Geometry: final body of the model. Coordinates: model frame, mm. A direction names the side the tool comes from. Give positions to 0.01 mm unless a question says otherwise; leave off trailing zeros. Write each loop counter-clockwise with the first axis right and the second up, starting at its lowest first coordinate (ties: lowest second). Pieces come first, ordered by that corner, then holes. Notation, with made-up numbers: M -37.5,-1 L -3.5,-1 A4 ccw -3.5,4 Z; hole C 53.5,-21.75 d1. An arc over 180 degrees is marked long. One line per question, with ' | ' between items.
from build123d import *

# Parameters (mm, degrees)
SKETCH1_W                   = 95.25
SKETCH1_H                   = 15
BOSS_EXTRUDE1_DEPTH         = 5
SKETCH2_W                   = 3
SKETCH2_H                   = 25.4
BOSS_EXTRUDE2_DEPTH         = 15
F_1_4_CLEARANCE_HOLE1_D     = 6.7564
F_1_4_CLEARANCE_HOLE1_DEPTH = 12
F_1_4_CLEARANCE_HOLE1_TIP   = 2.029827343
M3_CLEARANCE_HOLE1_D        = 3.6
M3_CLEARANCE_HOLE1_DEPTH    = 12
M3_CLEARANCE_HOLE1_TIP      = 1.081549114
CUT_EXTRUDE1_START          = -3
SKETCH9_R                   = 1.8
CUT_EXTRUDE1_DEPTH          = 3
FILLET1_R                   = 2
CHAMFER1_SIZE               = 1
CHAMFER2_SIZE               = 5
SKETCH10_W                  = 79.639400705
SKETCH10_H                  = 33.458041781
CUT_EXTRUDE2_DEPTH          = 57.020537529


with BuildPart() as part:
    # Sketch1 → Boss-Extrude1 (new body)
    with BuildSketch(Plane(origin=(0, 0, 0), x_dir=(1, 0, 0), z_dir=(0, 1, 0))):
        Rectangle(SKETCH1_W, SKETCH1_H)
    extrude(amount=BOSS_EXTRUDE1_DEPTH)

    # Sketch2 → Boss-Extrude2 (add, through all)
    with BuildSketch(Plane.XY.offset(7.5)):
        with Locations((-46.125, 12.7)):
            Rectangle(SKETCH2_W, SKETCH2_H)
    extrude(amount=-BOSS_EXTRUDE2_DEPTH)

    # 1/4 Clearance Hole1
    with Locations(Plane(origin=(-44.625, 0, 0), x_dir=(0, 0, -1), z_dir=(1, 0, 0))):
        with Locations((0, 12.7)):
            Hole(F_1_4_CLEARANCE_HOLE1_D / 2, depth=F_1_4_CLEARANCE_HOLE1_DEPTH)
            with Locations((0, 0, -(F_1_4_CLEARANCE_HOLE1_DEPTH + F_1_4_CLEARANCE_HOLE1_TIP / 2))):  # 118° drill point
                Cone(0, F_1_4_CLEARANCE_HOLE1_D / 2, F_1_4_CLEARANCE_HOLE1_TIP, mode=Mode.SUBTRACT)

    # M3 Clearance Hole1
    with Locations(Plane(origin=(0, 5, 0), x_dir=(1, 0, 0), z_dir=(0, 1, 0))):
        with Locations((-25, 0), (0, 0)):
            Hole(M3_CLEARANCE_HOLE1_D / 2, depth=M3_CLEARANCE_HOLE1_DEPTH)
            with Locations((0, 0, -(M3_CLEARANCE_HOLE1_DEPTH + M3_CLEARANCE_HOLE1_TIP / 2))):  # 118° drill point
                Cone(0, M3_CLEARANCE_HOLE1_D / 2, M3_CLEARANCE_HOLE1_TIP, mode=Mode.SUBTRACT)

    # Sketch9 → Cut-Extrude1 (cut)
    # profile 1 of 2: a face of its own
    with BuildSketch(Plane(origin=(0, 5, 0), x_dir=(1, 0, 0), z_dir=(0, 1, 0)).offset(CUT_EXTRUDE1_START)):
        with BuildLine():
            ThreePointArc((-26.670329309, -4.5), (-29.8, 0), (-26.670329309, 4.5))
            Line((-26.670329309, 4.5), (-41.625, 4.5))
            Line((-41.625, 4.5), (-41.625, -4.5))
            Line((-41.625, -4.5), (-26.670329309, -4.5))
        make_face()
    # profile 2 of 2: a face of its own
    with BuildSketch(Plane(origin=(0, 5, 0), x_dir=(1, 0, 0), z_dir=(0, 1, 0)).offset(CUT_EXTRUDE1_START)):
        with BuildLine():
            Line((44.625, -4.5), (44.625, 4.5))
            Line((44.625, 4.5), (-23.329670691, 4.5))
            ThreePointArc((-23.329670691, 4.5), (-21.059341382, 2.740658618), (-20.2, 0))
            ThreePointArc((-20.2, 0), (-21.059341382, -2.740658618), (-23.329670691, -4.5))
            Line((-23.329670691, -4.5), (44.625, -4.5))
        make_face()
        with Locations(Location((0, 0, 0), (0, 0, 270))):
            Circle(SKETCH9_R, mode=Mode.SUBTRACT)
    extrude(amount=CUT_EXTRUDE1_DEPTH, mode=Mode.SUBTRACT)

    # Fillet1
    fillet1_edges = [part.edges().sort_by_distance(p)[0] for p in [
        (-26.670329309, 3.5, -4.5),
        (-26.670329309, 3.5, 4.5),
        (-41.625, 3.5, 4.5),
        (-41.625, 3.5, -4.5),
        (-23.329670691, 3.5, 4.5),
        (-23.329670691, 3.5, -4.5),
    ]]
    fillet(fillet1_edges, radius=FILLET1_R)

    # Chamfer1
    chamfer1_edges = [part.edges().sort_by_distance(p)[0] for p in [
        (-44.625, 5, 0),
    ]]
    chamfer(chamfer1_edges, length=CHAMFER1_SIZE)

    # Chamfer2
    chamfer2_edges = [part.edges().sort_by_distance(p)[0] for p in [
        (-46.125, 25.4, 7.5),
        (-46.125, 25.4, -7.5),
    ]]
    chamfer(chamfer2_edges, length=CHAMFER2_SIZE)

    # Sketch10 → Cut-Extrude2 (cut, through all)
    with BuildSketch(Plane.XY.offset(7.5)):
        with Locations((39.819700352, 16.72902089)):
            Rectangle(SKETCH10_W, SKETCH10_H)
    extrude(amount=-CUT_EXTRUDE2_DEPTH, mode=Mode.SUBTRACT)

    # Mirror2: part across plane


with BuildPart() as part_1:
    add(part.part)
    add(part.part.mirror(Plane(origin=(0, 0, 0), x_dir=(0, 0, 1), z_dir=(1, 0, 0))))


solid = part_1.part
(1) Set-up query: faces 1 (the face through (-20, 4, 4)), 2 (the face through (-26.717, 2.465, -0.541)). Return all of +Z, -Z, +X, -X, +Y, -Y with unobstructed straight access to the full face (end or side cutting, diameter ignored); none if empty.
Working result:
face 1: +Y | face 2: +Y, -Y
(2) Cut plane B-B, the plane x = -25. Return loops of the section in (y, z), then the cut area to 3 significant figures.
Working result:
outline: M 0,-7.5 L 5,-7.5 L 5,-1.8 L 0,-1.8 Z; M 0,1.8 L 5,1.8 L 5,7.5 L 0,7.5 Z | area: 57.0 mm^2
(3) Material intervals for L1, parallel to X at y = 6, z = 4.25 (3 decimals); L2, parallel to Z at x = -25, y = 2.9; L3, parallel to Y at x = 46.35, z = 0, sorted ascending. Write a range as [from, to].
Working result:
L1: x = [-47.625, -44.625], [44.625, 47.625] | L2: z = [-7.5, -1.8], [1.8, 7.5] | L3: y = [0, 9.32], [16.08, 25.4]
(4) Cut plane A-A, the plane y = 4. Count the separate pieces of the cut face and the enclosed holes in it, then the cut area to 3 significant figures.
Working result:
separate pieces: 1 | enclosed holes: 5 | area: 831 mm^2
(5) Draft query along Y for faces 3 (the face through (46.15, 9.4, -0.73)), 4 (the face through (30, 4, -4)), 5 (the face through (-46.1, 22.9, 5)). Return one class per face: released by +Y, released by -Y, zero draft, split by the parting line, or undercut.
Working result:
face 3: undercut | face 4: zero draft | face 5: released by +Y
(6) Cut plane C-C, the plane y = 12.7. Return loops of the section in (x, z) (3 decimals), then the cut area to 3 significant figures.
Working result:
outline: M -47.625,-7.5 L -44.625,-7.5 L -44.625,-3.378 L -47.625,-3.378 Z; M -47.625,3.378 L -44.625,3.378 L -44.625,7.5 L -47.625,7.5 Z; M 44.625,-7.5 L 47.625,-7.5 L 47.625,-3.378 L 44.625,-3.378 Z; M 44.625,3.378 L 47.625,3.378 L 47.625,7.5 L 44.625,7.5 Z | area: 49.5 mm^2
(7) First-contact query: P1, Ø7, axis at x = -37.5, z = 0, coming from the +Y side; P2, Ø8, axis at x = 18.5, z = 3, coming from the +Y side. Flat tips, straight axial feed; report the tip coordinate or a pass-through.
Working result:
P1: stops at y = 2 | P2: stops at y = 5
(8) Cut plane D-D, the plane y = 7.75. Return loops of the section in (x, z) (3 decimals), then the cut area to 3 significant figures.
Working result:
outline: M -47.625,-7.5 L -44.625,-7.5 L -44.625,7.5 L -47.625,7.5 Z; M 44.625,-7.5 L 47.625,-7.5 L 47.625,7.5 L 44.625,7.5 Z | area: 90.0 mm^2
